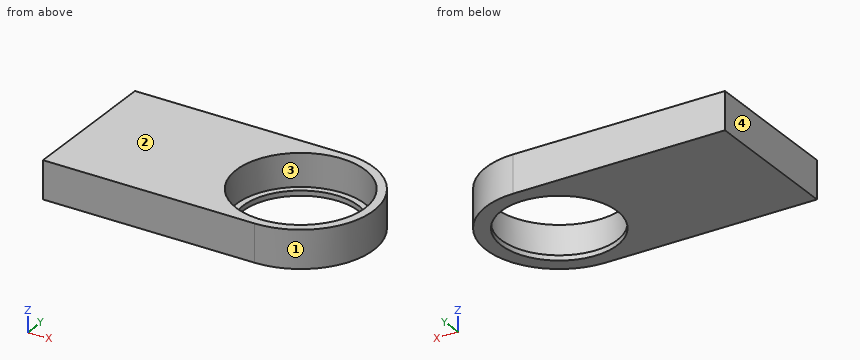
Autodesk Inventor part; units mm, degrees
ref_plane "YZ Plane" through (0, 0, 0) normal (1, 0, 0) x (0, 1, 0)
ref_plane "XZ Plane" through (0, 0, 0) normal (0, 1, 0) x (-1, 0, 0)
ref_plane "XY Plane" through (0, 0, 0) normal (0, 0, 1) x (1, 0, 0)
ref_plane "Work Plane1" through (0, 0, 0) normal (0, 0, 1) x (1, 0, 0)
sketch "Sketch1" plane through (0, 0, 0) normal (0, 0, 1) x (1, 0, 0)
  arc A0 (-18.155, 30) -> (-18.155, 0) centre (0, 15) ccw construction
  line L0 (-18.155, 0) -> (-3.4871, 0) construction
  line L1 (-18.155, 30) -> (-3.4871, 30) construction
  circle A1 centre (0, 15) radius 15.4 construction
  arc A2 (-6.5238, 29.5) -> (-6.5238, 0.5) centre (0, 15) ccw construction
  line L2 (-6.5238, 0.5) -> (-17.9179, 0.5) construction
  arc A3 (-17.9179, 29.5) -> (-17.9179, 0.5) centre (0, 15) ccw construction
  line L3 (-17.9179, 29.5) -> (-6.5238, 29.5) construction
  circle A4 centre (0, 15) radius 12.775 construction
  line L4 (-6.5238, 29.5) -> (0, 29.5) construction
  line L5 (-6.5238, 0.5) -> (0, 0.5) construction
  arc A5 (0, 0.5) -> (0, 29.5) centre (0, 15) ccw construction
  line L6 (-42.0841, 29.5) -> (-42.0841, 0.5)
  line L7 (-42.0841, 0.5) -> (0, 0.5)
  line L8 (-42.0841, 29.5) -> (0, 29.5)
  circle A6 centre (0, 15) radius 11.5
  arc A7 (0, 0.5) -> (0, 29.5) centre (0, 15) ccw
  arc A8 (-3.4871, 0) -> (3.4871, 0) centre (0, 15) ccw
  line L9 (3.4871, 0) -> (18, 0)
  line L10 (18, 0) -> (18, 30)
  line L11 (3.4871, 30) -> (18, 30)
  arc A9 (3.4871, 30) -> (-3.4871, 30) centre (0, 15) ccw
  line L12 (-7.3927, 28.5095) -> (7.3927, 28.5095)
  arc A10 (7.3927, 1.4905) -> (7.3927, 28.5095) centre (0, 15) ccw
  line L13 (7.3927, 1.4905) -> (-7.3927, 1.4905)
  arc A11 (-7.3927, 28.5095) -> (-7.3927, 1.4905) centre (0, 15) ccw
  point P0 (0, 0)
  dimension "d0" = 0.5
  dimension "d1" = 25.55
  dimension "d2" = 23
extrude "Extrusion1" add sketch "Sketch1" along normal blind 1 contours L8 A7 L12 A11 L13 L7 L6 | A7 L13 A11 L12
sketch "Sketch2" plane through (0, 0, 1) normal (0, 0, 1) x (1, 0, 0)
  circle A0 centre (0, 15) radius 11.5
  line L0 (0, 29.5) -> (-42.0841, 29.5)
  line L1 (-42.0841, 29.5) -> (-42.0841, 0.5)
  line L2 (-42.0841, 0.5) -> (0, 0.5)
  arc A1 (0, 0.5) -> (0, 29.5) centre (0, 15) ccw
  circle A2 centre (0, 15) radius 12.775
  point P0 (0, 0)
  dimension "d5" = 25.55
extrude "Extrusion2" add sketch "Sketch2" along normal blind 6.5 contours A1 L2 L1 L0
properties part number "10_Filteslide_25mm"
Verification items for the finished model (mm, model axes). Face numbers are marked on the shaded views. Give positions to 0.01 mm unless a question says otherwise; leave off trailing zeros. Loops run counter-clockwise (first coordinate to the right, second up) from the corner with the lowest first, then second, coordinate; pieces in that order, holes last. Notation, with made-up numbers: (7, -1.5) - (16, -1.5) arc R15 cw to (16, 16.5) - close; hole circle Ø11 at (88, 28). An arc over 180 degrees is marked (long way). Write item = value, one per line. Start each with the question number.
Q1. Cross-section at A-A, the plane y = 15. Enter the section's corners in (x, z) (3 decimals).
Q2. Mould release check, pull along X, two halves, no side actions. Record for the marked faces 1, 2, 3 and 4: released by +X, released by -X, zero draft, split by the parting line, or undercut.
Q3. Cross-section at B-B, the plane z = 6. Enter the section's corners in (x, y) (3 decimals), and give its area (3 significant figures).
Q4. Thickness scan on line 1 (Y direction, x = 0, z = 0.3); line 2 (Y direction, x = 0, z = 3.5) (3 decimals); line 3 (X direction, y = 10, z = 4.5). Record the ranges inside material, lowest first.
Q5. Depth check by flat-ended pin: P1, Ø2, axis at x = 3.5, z = 3, coming from the +Y side; P2, Ø1.5, axis at y = 22, z = 5.5, coming from the +X side; P3, Ø1, axis at y = 7.5, z = 4, coming from the +X side. Enter the tip coordinate at first touch or a pass-through.
Q6. Cross-section at C-C, the plane y = 5. Enter the section's corners in (x, z).
Answer key:
q1.outline = (-42.084, 0) - (-11.5, 0) - (-11.5, 1) - (-12.775, 1) - (-12.775, 7.5) - (-42.084, 7.5) - close; (11.5, 0) - (14.5, 0) - (14.5, 7.5) - (12.775, 7.5) - (12.775, 1) - (11.5, 1) - close
q2.face_1 = released by +X
q2.face_2 = zero draft
q2.face_3 = undercut
q2.face_4 = released by -X
q3.outline = (-42.084, 0.5) - (0, 0.5) arc R14.5 ccw to (0, 29.5) - (-42.084, 29.5) - close; hole circle Ø25.55 at (0, 15)
q3.area = 1,040 mm^2
q4.line_1 = 0.5 to 3.5, 26.5 to 29.5
q4.line_2 = 0.5 to 2.225, 27.775 to 29.5
q4.line_3 = -42.08 to -11.76, 11.76 to 13.61
q5.P1 = 29.28
q5.P2 = 13.08
q5.P3 = 12.7
q6.outline = (-42.08, 0) - (-5.68, 0) - (-5.68, 1) - (-7.95, 1) - (-7.95, 7.5) - (-42.08, 7.5) - close; (5.68, 0) - (10.5, 0) - (10.5, 7.5) - (7.95, 7.5) - (7.95, 1) - (5.68, 1) - close
